Could you check a few things on this drawing? It's one solid part, dimensions in mm from its lowest x, y, z. A direction names the side the tool comes from. Coordinates: 2 decimals unless noted, no trailing zeros. Order: outer loops, then holes, each group sorted by start corner. A loop starts at its lowest first (then second) coordinate and runs counter-clockwise, first axis right, second up. Notation, with made-up numbers: M 9.5,-11.5 L 34.5,-11.5 A26 cw 34.5,3.5 Z; hole C 88.5,3 d7. An arc over 180 degrees is marked long. Write item = value, one per line. Start each with the question number.
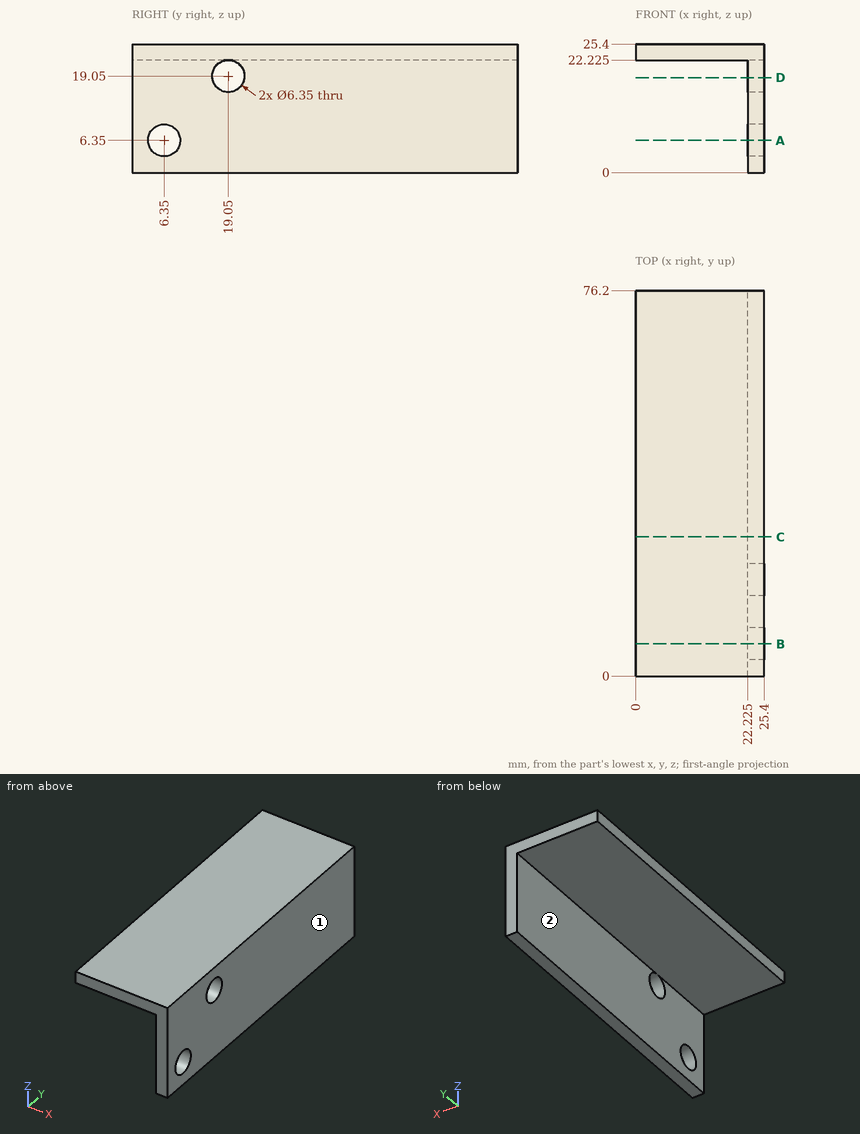
(1) For the marked faces 1 and 2, which set-ups out of +Z, -Z, +X, -X, +Y, -Y let a thin tool reach every point of the face, with its end or its side?
(2) Will these pins go through, and if not, where does the flat tip stop? P1, Ø1.5, axis at y = 23, z = 18, coming from the -X side (3 decimals); P2, Ø10, axis at x = 5.5, z = 15.5, coming from the -Y side; P3, Ø5, axis at x = 5.5, y = 15, coming from the -Z side (3 decimals).
(3) Please list where these lines run through material, in increasing order: probe 1 along Z at (x, y) = (22.9, 6.35) (3 decimals); probe 2 along Z at (x, y) = (23, 19.05) (3 decimals); probe 3 along Y at (x, z) = (23.9, 6.35) (3 decimals). Write a range as from..to.
(4) Imagine slicing it at B-B on y = 6.35. List the corners of the cut face in (x, z) for me (3 decimals).
(5) Imagine slicing it at C-C on y = 27.5. List the corners of the cut face in (x, z) for me (3 decimals).
(6) Imagine slicing it at A-A on z = 6.35. List the corners of the cut face in (x, y) for me (3 decimals), plus the area to 3 significant figures.
(7) Imagine slicing it at D-D on z = 18.75. List the corners of the cut face in (x, y) for me (3 decimals), plus the area to 3 significant figures.
Response:
q1.face_1 = +Z, -Z, +X, +Y, -Y
q1.face_2 = -Z, -X, +Y, -Y
q2.P1 = 22.225
q2.P2 = through
q2.P3 = 22.225
q3.probe_1 = 0..3.175, 9.525..25.4
q3.probe_2 = 0..15.875, 22.225..25.4
q3.probe_3 = 0..3.175, 9.525..76.2
q4.outline = M 0,22.225 L 22.225,22.225 L 22.225,9.525 L 25.4,9.525 L 25.4,25.4 L 0,25.4 Z; M 22.225,0 L 25.4,0 L 25.4,3.175 L 22.225,3.175 Z
q5.outline = M 0,22.225 L 22.225,22.225 L 22.225,0 L 25.4,0 L 25.4,25.4 L 0,25.4 Z
q6.outline = M 22.225,0 L 25.4,0 L 25.4,3.175 L 22.225,3.175 Z; M 22.225,9.525 L 25.4,9.525 L 25.4,76.2 L 22.225,76.2 Z
q6.area = 222 mm2
q7.outline = M 22.225,0 L 25.4,0 L 25.4,15.889 L 22.225,15.889 Z; M 22.225,22.211 L 25.4,22.211 L 25.4,76.2 L 22.225,76.2 Z
q7.area = 222 mm2
